Drawing for the job (mm, zero at the part's lowest x, y, z). A direction names the side the tool comes from. Give positions to 0.01 mm unless a question says otherwise; leave off trailing zeros. Loops run counter-clockwise (first coordinate to the right, second up) from the corner with the lowest first, then second, coordinate; pieces in that order, holes last. Notation, with made-up numbers: (45, 52) - (50, 52) arc R27 ccw to (50, 84) - close; hole circle Ø11 at (23, 56). An arc over 180 degrees is marked (long way). Return JSON: item names as keys, results as strings. Group by question number.
1) Slice it at C-C (x = 20). List the corners of the cut face in (y, z), and give its area (3 significant figures).
2) 3-axis set-ups, long thin cutter, end or side, ignore diameter. For the marked faces 4, 5 and 6: which of +Z, -Z, +X, -X, +Y, -Y reach the whole face in a straight line?
3) Drop flat-ended pins along their axis: pin 1 (1.5 mm diameter, centred on x = 21.5, y = 16.5, fed in from -Z); pin 2 (6 mm diameter, centred on x = 27, z = 32.5, fed in from +Y); pin 3 (6 mm diameter, centred on y = 123.5, z = 12, fed in from -X); pin 4 (2 mm diameter, centred on y = 54, z = 44.5, fed in from -X). Give the stop position or say it passes through.
4) Mould opens along Z. For the marked faces 1, 2 and 3 say: released by +Z, released by -Z, zero draft, split by the parting line, or undercut.
5) Slice it at D-D (z = 39.5). List the corners of the cut face in (x, y).
6) Slice it at A-A (z = 28). List the corners of the cut face in (x, y).
7) Slice it at B-B (y = 28). List the corners of the cut face in (x, z), and give its area (3 significant figures).
8) Drill centre lines: probe 1 along Y at (x, z) = (3, 28); probe 2 along X at (y, z) = (83, 16.5); probe 3 along Z at (x, y) = (30.5, 78). Where is each one in solid material? Low to high. Write a range as from..to.
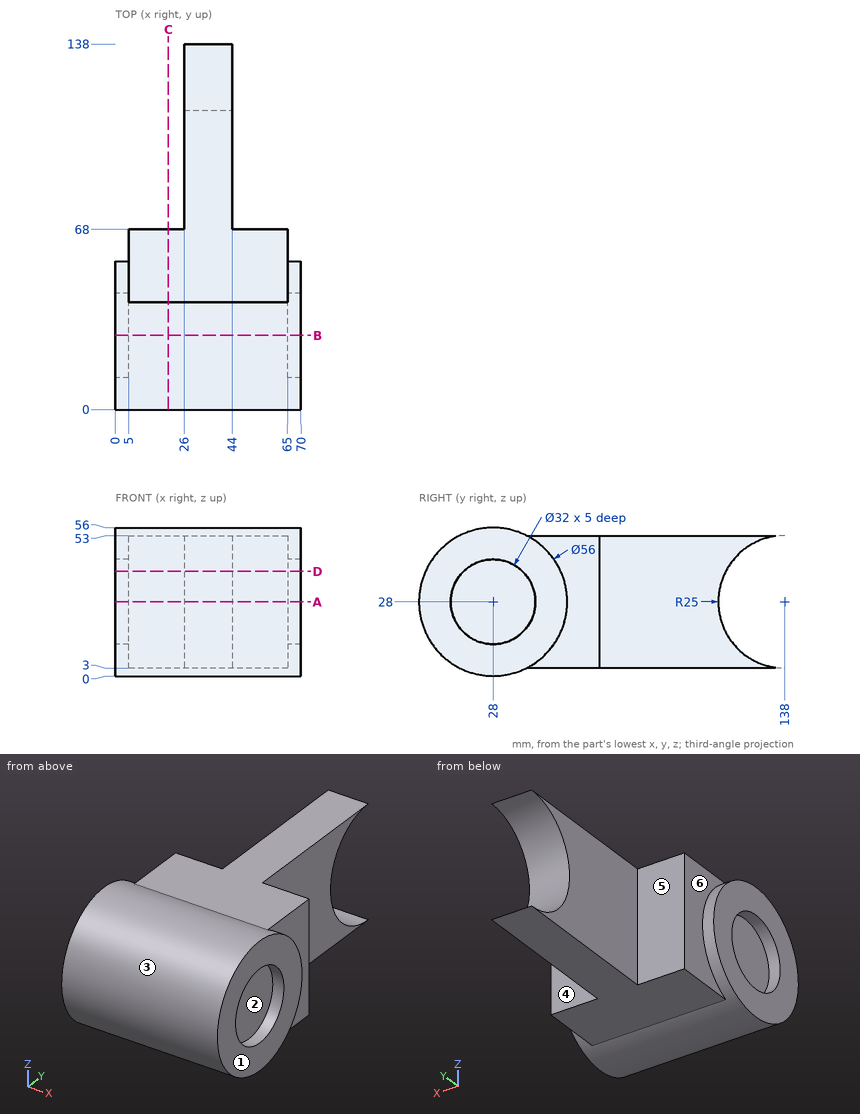
Results:
{
 "1": {"outline": "(40.61, 3) - (68, 3) - (68, 53) - (40.61, 53) arc R28 ccw (long way) to start", "area": "3,280 mm2"},
 "2": {"face 4": "+Z, -Z, +X, +Y", "face 5": "+Z, -Z, -X, +Y", "face 6": "-X, +Y"},
 "3": {"pin 1": "z = 2.15", "pin 2": "y = 114.15", "pin 3": "through", "pin 4": "x = 5"},
 "4": {"face 1": "zero draft", "face 2": "undercut", "face 3": "split by the parting line"},
 "5": {"outline": "(0, 2.47) - (70, 2.47) - (70, 16.88) - (65, 16.88) - (65, 39.12) - (70, 39.12) - (70, 53.53) - (65, 53.53) - (65, 68) - (44, 68) - (44, 115.8) - (26, 115.8) - (26, 68) - (5, 68) - (5, 53.53) - (0, 53.53) - (0, 39.12) - (5, 39.12) - (5, 16.88) - (0, 16.88) - close"},
 "6": {"outline": "(0, 0) - (70, 0) - (70, 12) - (65, 12) - (65, 44) - (70, 44) - (70, 56) - (65, 56) - (65, 68) - (44, 68) - (44, 113) - (26, 113) - (26, 68) - (5, 68) - (5, 56) - (0, 56) - (0, 44) - (5, 44) - (5, 12) - (0, 12) - close"},
 "7": {"outline": "(0, 0) - (70, 0) - (70, 12) - (65, 12) - (65, 44) - (70, 44) - (70, 56) - (0, 56) - (0, 44) - (5, 44) - (5, 12) - (0, 12) - close", "area": "3,600 mm2"},
 "8": {"probe 1": "0..12, 44..56", "probe 2": "26..44", "probe 3": "3..53"}
}
